Here's how the part is built. I have some questions about the finished solid (model axes, mm). A direction names the side the tool comes from. Give positions to 0.01 mm unless a question says otherwise; leave off trailing zeros. Write each loop counter-clockwise with the first axis right and the second up, starting at its lowest first coordinate (ties: lowest second). Pieces come first, ordered by that corner, then holes. Notation, with made-up numbers: (22, 46.25) - (69, 46.25) arc R15 cw to (69, 53.25) - close; hole circle Ø5 at (12, 3.5). An arc over 180 degrees is marked (long way). One line per item, written item: value. Start each with the question number.
1) On a 3-axis mill with a long thin cutter (end or side, diameter ignored), from which of +Z, -Z, +X, -X, +Y, -Y can I reach the whole of each face in a straight line? I mean faces 1 (the flat face through (-28, -23, -1.75)), 2 (the flat face through (-30, -13, -1.928)), 3 (the cylindrical face through (-25.922, 24.904, -3.144)), 4 (the flat face through (-31, 16.395, -6)). Say none if no direction works.
2) I'm going to push flat-ended pins straight in: P1, Ø3.5, axis at x = -28, y = -26, coming from the -Z side; P2, Ø2.5, axis at y = -10.5, z = 0.5, coming from the -X side; P3, Ø1.4, axis at x = -29.5, z = -1, coming from the -Y side; P4, Ø2, axis at x = -15, z = -2.5, coming from the +Y side. Where does each tip first touch, or does it pass through?
3) We'd pull the mould along X, two halves only. Please class faces 5 (the flat face through (-3.9, 24, -4)), 6 (the flat face through (40.5, 0, 4)), 7 (the flat face through (-32.82, 17.8, -5.6)), 8 (the flat face through (-30, -13, -3.4)): +X half, -X half, draft (parallel to the pull), parting line (faces both ways), or undercut.
4) Imagine slicing it at C-C on y = -4.5. Write out the boundary of the cut face in (x, z), plus the area to 3 significant figures.
5) Imagine slicing it at A-A on x = 10. Write out the boundary of the cut face in (y, z), plus the area to 3 significant figures.
6) Imagine slicing it at D-D on x = -6. Write out the boundary of the cut face in (y, z), plus the area to 3 significant figures.
7) Please list where these lines run through material, in increasing order: L1, parallel to Z at x = -30.5, y = 21; L2, parallel to Y at x = 20.5, z = -1; L3, parallel to Z at x = 9, y = -12.5. Write a range as [from, to].
8) Imagine slicing it at B-B on z = 2.5. Write out the boundary of the cut face in (x, y), plus the area to 3 significant figures.
from build123d import *

# Parameters (mm, degrees)
SKETCH1_W               = 81
SKETCH1_H               = 59.4
CARRIER_BASE_DEPTH      = 7.6
SKETCH2_W               = 7.7
SKETCH2_H               = 59.4
CUT_EXTRUDE1_DEPTH      = 4.8
SKETCH3_W               = 38.7
SKETCH3_H               = 2.5
ANALOG_POWER_BANK_DEPTH = 8.3
SKETCH4_W               = 37.2
SKETCH4_H               = 2.5
DIGITAL_BANK_DEPTH      = 8.3
SKETCH5_W               = 3.2
SKETCH5_H               = 8.8
F_5V_INPUT_DEPTH        = 11.3
SKETCH7_R               = 4.5
BOSS_EXTRUDE6_DEPTH     = 7.5
SKETCH8_R               = 3.019250474
CUT_EXTRUDE2_DEPTH      = 5
SKETCH9_W               = 6.4
SKETCH9_H               = 8.9
USB_C_DEPTH             = 3.4
FILLET3_R               = 0.5
CUT_EXTRUDE3_DEPTH      = 5.8
SKETCH11_W              = 6.5
SKETCH11_H              = 6.5
BOSS_EXTRUDE12_DEPTH    = 1.75
SKETCH12_R              = 1.697531851
RESET_DEPTH             = 1.75


with BuildPart() as part:
    # Sketch1 → Carrier / Base (new body)
    with BuildSketch(Plane.XY):
        Rectangle(SKETCH1_W, SKETCH1_H)
    extrude(amount=CARRIER_BASE_DEPTH)

    # Sketch2 → Cut-Extrude1 (cut)
    with BuildSketch(Plane(origin=(0, 0, 0), x_dir=(-1, 0, 0), z_dir=(0, 0, -1))):
        with Locations((36.65, 0)):
            Rectangle(SKETCH2_W, SKETCH2_H)
    extrude(amount=-CUT_EXTRUDE1_DEPTH, mode=Mode.SUBTRACT)

    # Sketch3 → Analog / Power Bank (add)
    with BuildSketch(Plane(origin=(0, 0, 0), x_dir=(-1, 0, 0), z_dir=(0, 0, -1))):
        with Locations((-15.45, 23.926979164)):
            Rectangle(SKETCH3_W, SKETCH3_H)
    extrude(amount=ANALOG_POWER_BANK_DEPTH)

    # Sketch4 → Digital Bank (add)
    with BuildSketch(Plane(origin=(0, 0, 0), x_dir=(-1, 0, 0), z_dir=(0, 0, -1))):
        with Locations((-19.6, -24.85)):
            Rectangle(SKETCH4_W, SKETCH4_H)
    extrude(amount=DIGITAL_BANK_DEPTH)

    # Sketch5 → 5V Input (add)
    with BuildSketch(Plane(origin=(0, 0, 0), x_dir=(-1, 0, 0), z_dir=(0, 0, -1))):
        with Locations((31.21956927, 20.79458393)):
            Rectangle(SKETCH5_W, SKETCH5_H)
    extrude(amount=F_5V_INPUT_DEPTH)

    # Sketch7 → Boss-Extrude6 (add)
    with BuildSketch(Plane(origin=(-29.61956927, 0, 0), x_dir=(0, 0, -1), z_dir=(1, 0, 0))):
        with Locations(Location((4.827826856, 20.730910649, 0), (0, 0, 254.499508307))):
            Circle(SKETCH7_R)
    extrude(amount=BOSS_EXTRUDE6_DEPTH)

    # Sketch8 → Cut-Extrude2 (cut)
    with BuildSketch(Plane.ZY.offset(32.81956927)):
        with Locations((-5.241560024, 20.985277651)):
            Circle(SKETCH8_R)
    extrude(amount=-CUT_EXTRUDE2_DEPTH, mode=Mode.SUBTRACT)

    # Sketch9 → USB-C (add)
    with BuildSketch(Plane(origin=(0, 0, 0), x_dir=(-1, 0, 0), z_dir=(0, 0, -1))):
        with Locations((29.6, -13.15)):
            Rectangle(SKETCH9_W, SKETCH9_H)
    extrude(amount=USB_C_DEPTH)

    # Fillet3
    fillet3_edges = [part.edges().sort_by_distance(p)[0] for p in [
        (-32.8, -13.15, -3.4),
        (-29.6, -8.7, -3.4),
        (-26.4, -13.15, -3.4),
        (-29.6, -17.6, -3.4),
    ]]
    fillet(fillet3_edges, radius=FILLET3_R)

    # Sketch10 → Cut-Extrude3 (cut)
    with BuildSketch(Plane.ZY.offset(32.8)):
        with BuildLine():
            Line((-1.928214934, -16.631364992), (-1.928214934, -9.789588696))
            ThreePointArc((-1.928214934, -9.789588696), (-1.229070102, -9.090443863), (-0.52992527, -9.789588696))
            Line((-0.52992527, -9.789588696), (-0.52992527, -16.631364992))
            ThreePointArc((-0.52992527, -16.631364992), (-1.229070102, -17.330509824), (-1.928214934, -16.631364992))
        make_face()
    extrude(amount=-CUT_EXTRUDE3_DEPTH, mode=Mode.SUBTRACT)

    # Sketch11 → Boss-Extrude12 (add)
    with BuildSketch(Plane(origin=(0, 0, 0), x_dir=(-1, 0, 0), z_dir=(0, 0, -1))):
        with Locations((27.822665658, -24.892209285)):
            Rectangle(SKETCH11_W, SKETCH11_H)
    extrude(amount=BOSS_EXTRUDE12_DEPTH)

    # Sketch12 → Reset (add)
    with BuildSketch(Plane(origin=(0, 0, -1.75), x_dir=(-1, 0, 0), z_dir=(0, 0, -1))):
        with Locations(Location((27.87525987, -25.172094467, 0), (0, 0, 180))):
            Circle(SKETCH12_R)
    extrude(amount=RESET_DEPTH)


solid = part.part
Numbers:
1. face 1: -Z
1. face 2: -X
1. face 3: none
1. face 4: -Z, -X
2. P1: z = -3.5
2. P2: x = -32.8
2. P3: y = -28.14
2. P4: through
3. face 5: undercut
3. face 6: +X half
3. face 7: -X half
3. face 8: draft
4. outline: (-40.5, 4.8) - (-32.8, 4.8) - (-32.8, 0) - (40.5, 0) - (40.5, 7.6) - (-40.5, 7.6) - close
4. area: 579 mm^2
5. outline: (-29.7, 0) - (-26.1, 0) - (-26.1, -8.3) - (-23.6, -8.3) - (-23.6, 0) - (22.68, 0) - (22.68, -8.3) - (25.18, -8.3) - (25.18, 0) - (29.7, 0) - (29.7, 7.6) - (-29.7, 7.6) - close
5. area: 493 mm^2
6. outline: (-29.7, 0) - (29.7, 0) - (29.7, 7.6) - (-29.7, 7.6) - close
6. area: 451 mm^2
7. L1: [-11.3, -8.26], [-2.22, 7.6]
7. L2: [-26.1, -23.6], [22.68, 25.18]
7. L3: [0, 7.6]
8. outline: (-32.8, -29.7) - (40.5, -29.7) - (40.5, 29.7) - (-32.8, 29.7) - close
8. area: 4,350 mm^2
